Part print with two shaded views. Sizes in mm from the minimum x, y, z corner. A direction names the side the tool comes from. Round coordinates to 2 decimals unless told otherwise and drop trailing zeros. Loops run counter-clockwise (first coordinate to the right, second up) from the corner with the lowest first, then second, coordinate; pieces in that order, holes last.
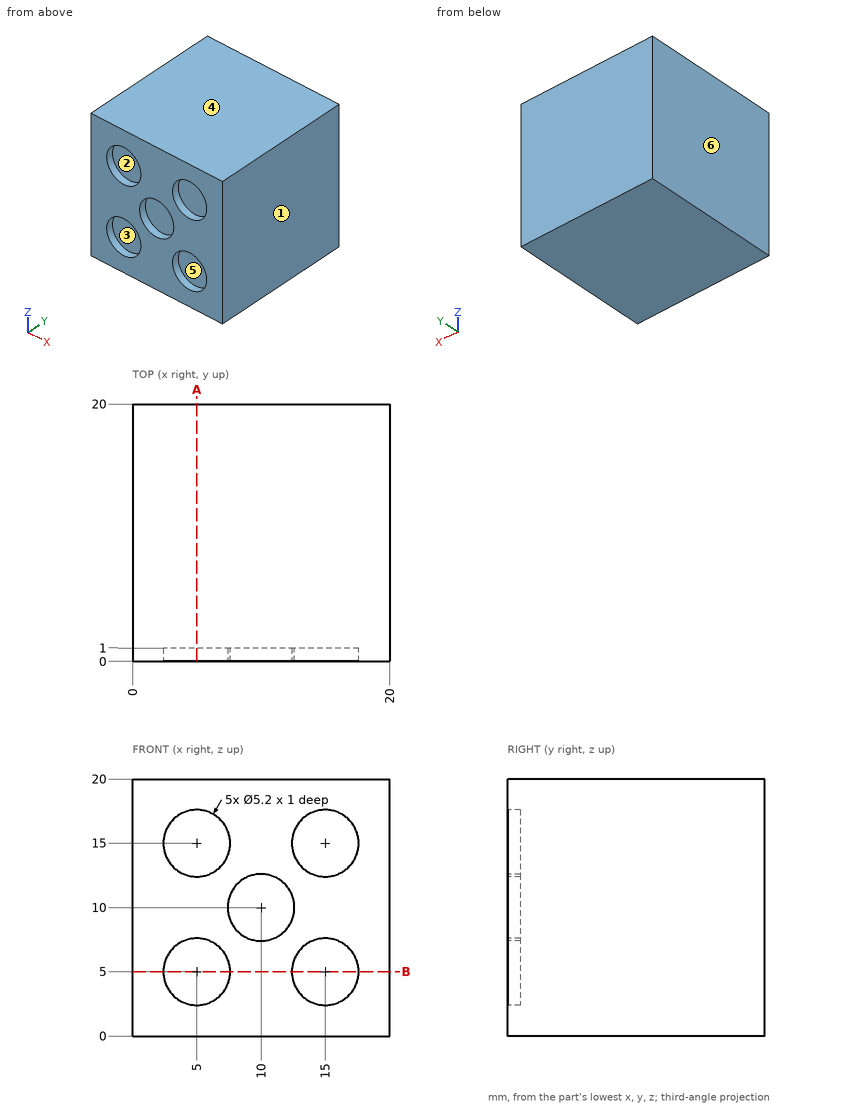
Item 1: Mould opens along Z. For the marked faces 3, 4, 5 and 6 say: released by +Z, released by -Z, zero draft, split by the parting line, or undercut.
Verdict:
face 3: undercut
face 4: released by +Z
face 5: undercut
face 6: zero draft
Item 2: Wall check: L1, parallel to Z at x = 15, y = 0.6; L2, parallel to Y at x = 14.5, z = 15.5. Give the ranges that are in metal, low to high.
Verdict:
L1: z = 0 to 2.4, 7.6 to 12.4, 17.6 to 20
L2: y = 1 to 20
Item 3: 3-axis set-ups, long thin cutter, end or side, ignore diameter. For the marked faces 1 and 2: which of +Z, -Z, +X, -X, +Y, -Y reach the whole face in a straight line?
Verdict:
face 1: +Z, -Z, +X, +Y, -Y
face 2: -Y
Item 4: Cut at B-B (z = 5). List the corners of the cut face in (x, y).
Verdict:
outline: (0, 0) - (2.4, 0) - (2.4, 1) - (7.6, 1) - (7.6, 0) - (12.4, 0) - (12.4, 1) - (17.6, 1) - (17.6, 0) - (20, 0) - (20, 20) - (0, 20) - close
Item 5: Flat gauge pin, fed straight in: P1, Ø3, axis at x = 15, z = 5, coming from the -Y side. Where does the tip first touch, or does it go through?
Verdict:
P1: stops at y = 1
Item 6: Cut at A-A (x = 5). List the corners of the cut face in (y, z), plus the area to 3 significant figures.
Verdict:
outline: (0, 0) - (20, 0) - (20, 20) - (0, 20) - (0, 17.6) - (1, 17.6) - (1, 12.4) - (0, 12.4) - (0, 7.6) - (1, 7.6) - (1, 2.4) - (0, 2.4) - close
area: 390 mm2
